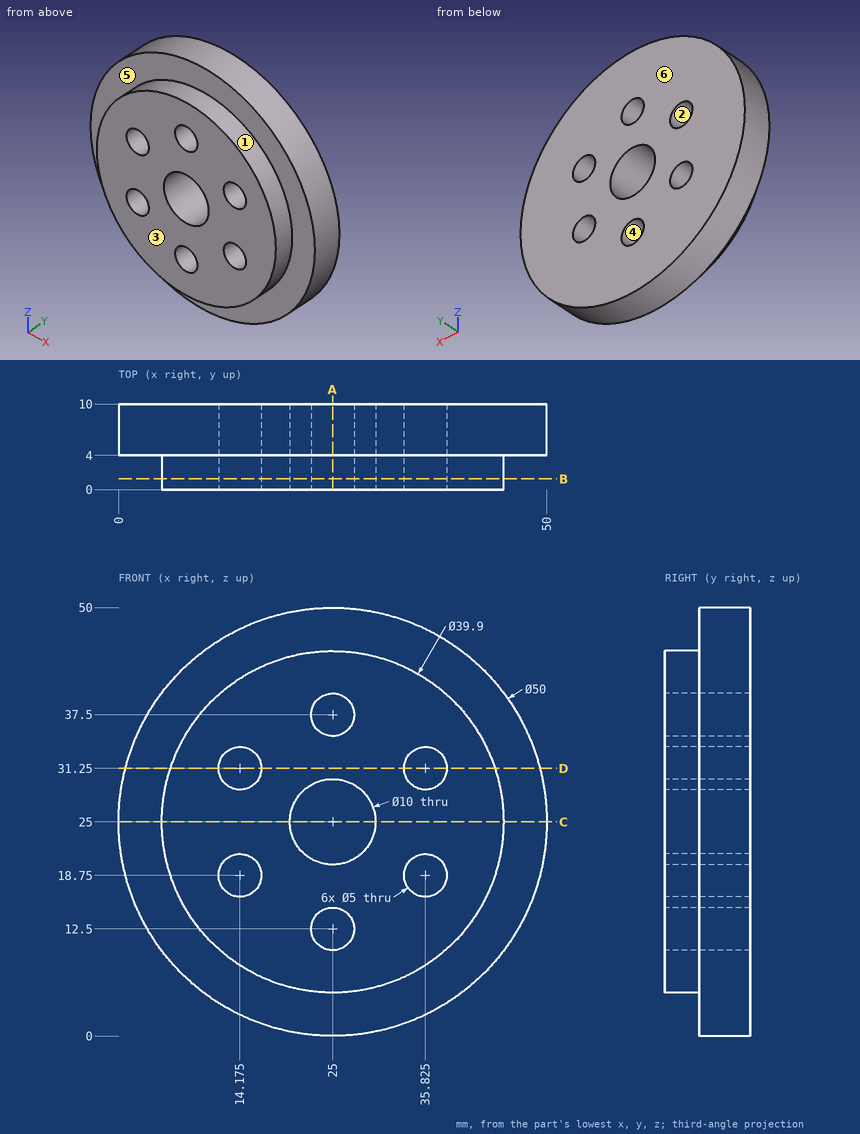
Could you check a few things on this drawing? It's one solid part, dimensions in mm from its lowest x, y, z. A direction names the side the tool comes from. Give positions to 0.01 mm unless a question says otherwise; leave off trailing zeros. Order: outer loops, then holes, each group sorted by start corner. A loop starts at its lowest first (then second) coordinate and runs counter-clockwise, first axis right, second up. Notation, with made-up numbers: M -21,18 L -10,18 A26 cw -10,54 Z; hole C -2.5,65.5 d2. An arc over 180 degrees is marked long. Use one line per item in the form item = value.
Item 1: For the marked faces 5 and 6, which set-ups out of +Z, -Z, +X, -X, +Y, -Y let a thin tool reach every point of the face, with its end or its side?
Values follow:
face_5 = -Y
face_6 = +Z, -Z, +X, -X, +Y
Item 2: If we section it at C-C, the plane z = 25: Write out the boundary of the cut face in (x, y).
Values follow:
outline = M 0,4 L 5.05,4 L 5.05,0 L 20,0 L 20,10 L 0,10 Z; M 30,0 L 44.95,0 L 44.95,4 L 50,4 L 50,10 L 30,10 Z
Item 3: If I drill on line 1 along X through (y, z) = (5, 25); line 2 along X through (y, z) = (3, 25); line 3 along X through (y, z) = (7.5, 19), over which ranges is the centre line in solid material (lowest first)? Write a range as [from, to].
Values follow:
line_1 = [0, 20], [30, 50]
line_2 = [5.05, 20], [30, 44.95]
line_3 = [0.73, 11.69], [16.66, 33.34], [38.31, 49.27]
Item 4: If we section it at D-D, the plane z = 31.25: Write out the boundary of the cut face in (x, y) (1 decimal).
Values follow:
outline = M 0.8,4 L 6.1,4 L 6.1,0 L 11.7,0 L 11.7,10 L 0.8,10 Z; M 16.7,0 L 33.3,0 L 33.3,10 L 16.7,10 Z; M 38.3,0 L 43.9,0 L 43.9,4 L 49.2,4 L 49.2,10 L 38.3,10 Z
Item 5: Will these pins go through, and if not, where does the flat tip stop? pin 1 Ø5 at (x, y) = (7.5, 6.5) entering from +Z; pin 2 Ø15 at (x, z) = (19.5, 31) entering from -Y; pin 3 Ø4 at (x, z) = (25, 37.5) entering from +Y; pin 4 Ø2 at (x, y) = (7, 8) entering from -Z.
Values follow:
pin_1 = 45
pin_2 = 0
pin_3 = through
pin_4 = 6.67
Item 6: If we section it at B-B, the plane y = 1.25: Count the separate pieces of the cut face and the enclosed holes in it, and give its area (3 significant figures).
Values follow:
separate_pieces = 1
enclosed_holes = 7
area = 1,050 mm^2
Item 7: Thinking about a two-plate mould opening in X: for the marked faces 1, 2, 3 and 4, which applies, pulls with the +X half, pulls with the -X half, needs draft (parallel to the pull), parting line crosses it, or undercut?
Values follow:
face_1 = parting line crosses it
face_2 = undercut
face_3 = needs draft
face_4 = undercut
Item 8: If we section it at A-A, the plane x = 25: Write out the boundary of the cut face in (y, z).
Values follow:
outline = M 0,5.05 L 4,5.05 L 4,0 L 10,0 L 10,10 L 0,10 Z; M 0,15 L 10,15 L 10,20 L 0,20 Z; M 0,30 L 10,30 L 10,35 L 0,35 Z; M 0,40 L 10,40 L 10,50 L 4,50 L 4,44.95 L 0,44.95 Z
